For this review, take the finished solid that the model builds, in its own axes (mm). A direction names the side the tool comes from. Round coordinates to 2 decimals unless told otherwise and drop trailing zeros. Order: outer loops, then holes, each group sorted by start corner. A loop starts at its lowest first (then second) coordinate and runs counter-clockwise, first axis right, second up. Notation, with made-up numbers: M 63.5,-26.5 L 74.5,-26.5 A8 cw 74.5,-11.5 Z; hole C 25,-3 d6. An arc over 180 degrees is marked long. Write item = value, one per line. Start each with the question number.
Autodesk Inventor part; units mm, degrees
ref_plane "YZ Plane" through (0, 0, 0) normal (1, 0, 0) x (0, 1, 0)
ref_plane "XZ Plane" through (0, 0, 0) normal (0, 1, 0) x (-1, 0, 0)
ref_plane "XY Plane" through (0, 0, 0) normal (0, 0, 1) x (1, 0, 0)
sketch "Sketch1" plane through (0, 0, 0) normal (0, 0, 1) x (1, 0, 0)
  line L0 (-4.25, 4.25) -> (4.25, 4.25)
  line L1 (4.25, 4.25) -> (4.25, -4.25)
  line L2 (4.25, -4.25) -> (-4.25, -4.25)
  line L3 (-4.25, -4.25) -> (-4.25, 4.25)
  point P0 (0, 0)
  dimension "d0" = 8.5
  dimension "d1" = 8.5
  dimension "d2" = 4.25
  dimension "d3" = 4.25
extrude "Extrusion1" add sketch "Sketch1" along normal blind 2.5
fillet "Fillet2" radius 1 3 edges at (4.25, 4.25, 1.25) (4.25, 0, 0) (0, 4.25, 0)
sketch "Sketch10" plane through (0, 0, 2.5) normal (0, 0, 1) x (1, 0, 0)
  line L0 (4.25, 3.25) -> (4.25, -4.25)
  line L1 (-4.25, 4.25) -> (3.25, 4.25)
  line L2 (3.25, 3.25) -> (-17.75, 3.25)
  line L3 (-17.75, 3.25) -> (-17.75, -17.75)
  line L4 (-17.75, -17.75) -> (3.25, -17.75)
  line L5 (3.25, -17.75) -> (3.25, 3.25)
  point P0 (0, 0)
  dimension "d113" = 1
  dimension "d114" = 1
  dimension "d115" = 21
  dimension "d116" = 21
extrude "Extrusion8" add sketch "Sketch10" along normal blind 7
hole "Hole9" at (3.25, -7.75, 6.5) direction (-1, 0, 0) diameter 2.3876 depth 5 tip angle 118 countersink diameter 2.54 countersink angle 120
hole "Hole10" at (-7.75, 3.25, 6.5) direction (0, -1, 0) diameter 2.3876 depth 5 tip angle 118 countersink diameter 2.54 countersink angle 120
hole "Hole11" at (-6.25, -6.25, 9.5) direction (0, 0, -1) diameter 6.35 depth 5
sketch "Sketch11" plane through (0, 0, 2.5) normal (0, 0, -1) x (-1, 0, 0)
  line L0 (17.75, -17.75) -> (-3.25, -17.75)
  line L1 (17.75, 3.25) -> (17.75, -17.75)
  line L2 (4.25, 3.25) -> (17.75, 3.25)
  line L3 (10.75, 3.25) -> (17.75, 3.25)
  line L4 (17.75, 3.25) -> (17.75, -17.75)
  line L5 (17.75, -17.75) -> (-3.25, -17.75)
  line L6 (-3.25, -17.75) -> (-3.25, -10.75)
  line L7 (-3.25, -10.75) -> (0.75, -10.75)
  line L8 (0.75, -10.75) -> (10.75, -0.75)
  line L9 (10.75, -0.75) -> (10.75, 3.25)
  point P0 (0, 0)
  dimension "d146" = 14
  dimension "d158" = 4
extrude "Extrusion9" cut sketch "Sketch11" against normal blind 3.325
hole "Hole12" at (-0.25, -14.75, 5.825) direction (0, 0, 1) diameter 2.3876 end through all countersink diameter 2.54 countersink angle 120
hole "Hole13" at (-14.75, -0.25, 5.825) direction (0, 0, 1) diameter 2.3876 end through all countersink diameter 2.54 countersink angle 120
chamfer "Chamfer3" distance 16 angle 45 1 edges at (-17.75, -17.75, 7.6625)
chamfer "Chamfer4" distance 1 angle 45 2 edges at (-7.25, 3.25, 9.5) (3.25, -7.25, 9.5)
sketch "Sketch15" plane through (0, 0, 2.5) normal (0, 0, 1) x (1, 0, 0)
  line L0 (-4.25, 3.25) -> (3.25, 3.25)
  line L1 (3.25, 3.25) -> (3.25, -4.25)
  line L2 (4.25, -4.25) -> (3.25, -4.25)
  line L3 (4.25, 3.25) -> (4.25, -4.25)
  arc A0 (4.25, 3.25) -> (3.25, 4.25) centre (3.25, 3.25) ccw
  line L4 (-4.25, 4.25) -> (3.25, 4.25)
  line L5 (-4.25, 3.25) -> (-4.25, 4.25)
  point P0 (0, 0)
extrude "Extrusion11" [suppressed]
chamfer "Chamfer6" distance 1 angle 45 1 edges at (3.25, 3.25, 5.5)
hole "Hole16" at (-0.5, -0.5, 0) direction (0, 0, 1) diameter 3.4544 end through all countersink diameter 4.064 countersink angle 120
sketch "Sketch16" plane through (0, 0, 2.5) normal (0, 0, -1) x (-1, 0, 0)
  line L0 (-3.25, -10.75) -> (0.75, -10.75)
  line L1 (10.75, -0.75) -> (10.75, 3.25)
  line L2 (4.25, 3.25) -> (10.75, 3.25)
  line L3 (4.25, -4.25) -> (4.25, 3.25)
  line L4 (-3.25, -4.25) -> (4.25, -4.25)
  line L5 (-3.25, -10.75) -> (-3.25, -4.25)
  line L6 (4.25, 4.25) -> (10.75, 4.25)
  line L7 (10.75, 4.25) -> (10.75, -0.75)
  line L8 (10.75, -0.75) -> (0.75, -10.75)
  line L9 (0.75, -10.75) -> (-4.25, -10.75)
  line L10 (-4.25, -10.75) -> (-4.25, -4.25)
  line L11 (-4.25, -4.25) -> (4.25, -4.25)
  line L12 (4.25, -4.25) -> (4.25, 4.25)
  point P0 (0, 0)
  dimension "d213" = 1
  dimension "d214" = 1
extrude "Extrusion12" add sketch "Sketch16" along normal blind 1
properties part number "FOX-ME-121-03" material "Aluminum-6061"
(1) For line 1 along X through (y, z) = (-0.5, 4.5); line 2 along X through (y, z) = (1, 6.5); line 3 along Z through (x, y) = (-7.75, 2), list the stretches that pass through material, from the lowest coordinate up.
(2) Draft analysis for pull direction Z (two halves, no side actions). For faces 4 (the flat face through (4.25, -4, 2)), 5 (the flat face through (2.74, -7.36, 9.01)), 6 (the conical face through (-2.343, -7.575, 6.389)), state which applies: released by +Z, released by -Z, zero draft, split by the parting line, or undercut.
(3) We need section A-A, the plane y = -14.75. Write out the cut boundary in (x, z) (3 decimals), then the cut area to 3 significant figures.
(4) We need section C-C, the plane x = -11.5. Write out the cut boundary in (y, z) (3 decimals), then the cut area to 3 significant figures.
(5) We need section D-D, the plane y = -0.25. State how many separate pieces and enclosed holes the cut face has, then the cut area to 3 significant figures.
(6) We need section B-B, the plane z = 4. Write out the cut boundary in (x, y).
(7) For faces 1 (the flat face through (-7, -10, 5.825)), 2 (the flat face through (0, 3.5, 2.5)), 3 (the flat face through (0, -4.25, 1)), list the 3-axis set-ups (+Z, -Z, +X, -X, +Y, -Y) from which the entire face can be reached by the end or side of a thin tool; tool diameter is ignored.
(8) Insertion check: pin 1 (2 mm diameter, centred on x = -0.25, y = -14.75, fed in from -Z); pin 2 (1.6 mm diameter, centred on y = 0, z = 0.5, fed in from -X); pin 3 (1.9 mm diameter, centred on x = -7.75, z = 6.5, fed in from +Y); pin 4 (4 mm diameter, centred on x = -12, z = 4, fed in from -Y). Each pin has a flat end and moves straight along its axis. Give the tip position at first contact, or say it passes through.
Values:
q1.line_1 = -10.75 to -2.23, 1.23 to 3.25
q1.line_2 = -17.75 to -8.94, -6.56 to -1.36, 0.36 to 3.25
q1.line_3 = 1.5 to 5.31, 7.69 to 9.5
q2.face_4 = zero draft
q2.face_5 = released by +Z
q2.face_6 = undercut
q3.outline = M -4.75,5.825 L -1.52,5.825 L -1.444,5.869 L -1.444,9.5 L -4.75,9.5 Z; M 0.944,5.869 L 1.02,5.825 L 3.25,5.825 L 3.25,8.5 L 2.25,9.5 L 0.944,9.5 Z
q3.area = 20.1 mm²
q4.outline = M -8,5.825 L 3.25,5.825 L 3.25,8.5 L 2.25,9.5 L -8,9.5 Z
q4.area = 40.8 mm²
q5.separate_pieces = 3
q5.enclosed_holes = 1
q5.area = 105 mm²
q6.outline = M -10.75,-0.75 L -0.75,-10.75 L 3.25,-10.75 L 3.25,2.25 L 2.25,3.25 L -10.75,3.25 Z; hole C -0.5,-0.5 d3.45
q7.face_1 = -Z, -X, -Y
q7.face_2 = +Z, +X, +Y
q7.face_3 = -Z, +X, -X, -Y
q8.pin_1 = through
q8.pin_2 = -4.25
q8.pin_3 = -1.9
q8.pin_4 = -8.32
